```python
from build123d import *

# Parameters (mm, degrees)
SKETCH_1_W      = 7
SKETCH_1_H      = 17
SKETCH_1_W_2    = 8
SKETCH_1_H_2    = 3
EXTRUDE_1_DEPTH = 3
FILLET_1_R      = 0.5


with BuildPart() as part:
    # 草图1 → 凸台-拉伸1 (new body)
    # profile 1 of 5: a face of its own
    with BuildSketch(Plane(origin=(0, 0, 0), x_dir=(1, 0, 0), z_dir=(0, 1, 0))):
        Polygon((-4, 17), (-7, 17), (-7, -17), (-4, -17), (-4, -14), (4, -14), (4, -17), (7, -17), (7, 17), (4, 17), (4, 14), (-4, 14), align=None)
        Rectangle(SKETCH_1_W, SKETCH_1_H, mode=Mode.SUBTRACT)
    # profile 2 of 5: a face of its own
    with BuildSketch(Plane(origin=(0, 0, 0), x_dir=(1, 0, 0), z_dir=(0, 1, 0))):
        with Locations((0, 18.5)):
            Rectangle(SKETCH_1_W_2, SKETCH_1_H_2)
    # profile 3 of 5: a face of its own
    with BuildSketch(Plane(origin=(0, 0, 0), x_dir=(1, 0, 0), z_dir=(0, 1, 0))):
        with Locations((0, 15.5)):
            Rectangle(SKETCH_1_W_2, SKETCH_1_H_2)
    # profile 4 of 5: a face of its own
    with BuildSketch(Plane(origin=(0, 0, 0), x_dir=(1, 0, 0), z_dir=(0, 1, 0))):
        with Locations((0, -18.5)):
            Rectangle(SKETCH_1_W_2, SKETCH_1_H_2)
    # profile 5 of 5: a face of its own
    with BuildSketch(Plane(origin=(0, 0, 0), x_dir=(1, 0, 0), z_dir=(0, 1, 0))):
        with Locations((0, -15.5)):
            Rectangle(SKETCH_1_W_2, SKETCH_1_H_2)
    extrude(amount=EXTRUDE_1_DEPTH)

    # 圆角1
    fillet_1_edges = [part.edges().sort_by_distance(p)[0] for p in [
        (-3.5, 1.5, -8.5),
        (-3.5, 1.5, 8.5),
        (3.5, 1.5, 8.5),
        (3.5, 1.5, -8.5),
        (-4, 1.5, -17),
        (4, 1.5, -17),
        (4, 1.5, 17),
        (-4, 1.5, 17),
    ]]
    fillet(fillet_1_edges, radius=FILLET_1_R)


solid = part.part
```
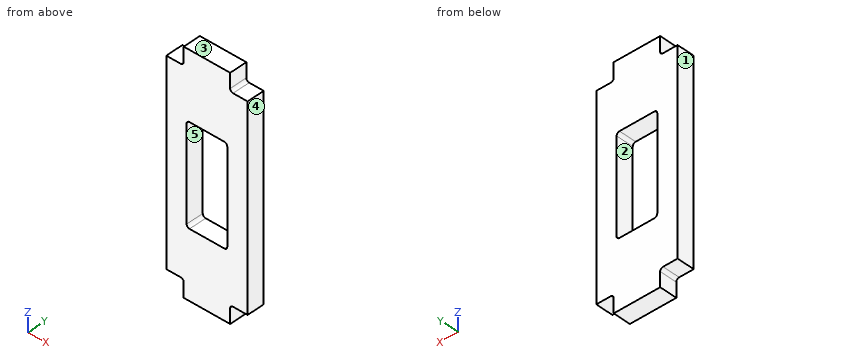
Model file for the job. Use its own axes, mm. Face numbers are marked on the shaded views. A direction names the side the tool comes from. Coordinates: 2 decimals unless noted, no trailing zeros. Loops run counter-clockwise (first coordinate to the right, second up) from the corner with the lowest first, then second, coordinate; pieces in that order, holes last. Notation, with made-up numbers: (-32.75, 49) - (-2.75, 49) arc R35 ccw to (-2.75, 81) - close; hole circle Ø7 at (-12.5, -20.5). An arc over 180 degrees is marked (long way). Answer as a JSON object with one key per item and string values. Group by question number.
(1) Cut at B-B (x = 2.5). Give the cut face in (y, z).
(2) Cut at D-D (x = 5). Give the cut face in (y, z).
(3) Probe line 1 along X through (y, z) = (0.95, -8); line 2 along Z through (x, y) = (1, 1.15); line 3 along Z through (x, y) = (4.5, 2). List the from-to ranges inside material, lowest first.
(4) Two-plate mould, pull along X, no slides. Class the marked faces 1, 2 and 3: released by +X, released by -X, zero draft, split by the parting line, or undercut.
(5) Cut at C-C (y = 1.1). Give the cut face in (x, z).
(6) Flat gauge pins, fed straight in: pin 1 (1.2 mm diameter, centred on y = 1, z = -18.5, fed in from -X); pin 2 (3 mm diameter, centred on x = 1, z = -6, fed in from -Y); pin 3 (0.8 mm diameter, centred on x = -6, y = 1.5, fed in from -Z); pin 4 (0.8 mm diameter, centred on x = 5, y = 2, fed in from +Z). Where does each tip first touch, or does it go through?
(7) Cut at A-A (z = 6.5). Give the cut face in (x, y), then the cut area to 3 significant figures.
(8) Tool access for the marked faces 4 and 5: list every direction of +Z, -Z, +X, -X, +Y, -Y with a clear straight run to the whole face (end or side of a thin tool).
Geometry says:
{
 "1": {"outline": "(0, -20) - (3, -20) - (3, -8.5) - (0, -8.5) - close; (0, 8.5) - (3, 8.5) - (3, 20) - (0, 20) - close"},
 "2": {"outline": "(0, -17) - (3, -17) - (3, 17) - (0, 17) - close"},
 "3": {"line 1": "x = -7 to -3.5, 3.5 to 7", "line 2": "z = -20 to -8.5, 8.5 to 20", "line 3": "z = -17 to 17"},
 "4": {"face 1": "released by -X", "face 2": "undercut", "face 3": "zero draft"},
 "5": {"outline": "(-7, -17) - (-4.5, -17) arc R0.5 cw to (-4, -17.5) - (-4, -20) - (4, -20) - (4, -17.5) arc R0.5 cw to (4.5, -17) - (7, -17) - (7, 17) - (4.5, 17) arc R0.5 cw to (4, 17.5) - (4, 20) - (-4, 20) - (-4, 17.5) arc R0.5 cw to (-4.5, 17) - (-7, 17) - close; hole (-3.5, -8) arc R0.5 ccw to (-3, -8.5) - (3, -8.5) arc R0.5 ccw to (3.5, -8) - (3.5, 8) arc R0.5 ccw to (3, 8.5) - (-3, 8.5) arc R0.5 ccw to (-3.5, 8) - close"},
 "6": {"pin 1": "stops at x = -4", "pin 2": "passes through", "pin 3": "stops at z = -17", "pin 4": "stops at z = 17"},
 "7": {"outline": "(-7, 0) - (-3.5, 0) - (-3.5, 3) - (-7, 3) - close; (3.5, 0) - (7, 0) - (7, 3) - (3.5, 3) - close", "area": "21.0 mm^2"},
 "8": {"face 4": "+Z, -Z, +X, +Y, -Y", "face 5": "+Y, -Y"}
}
